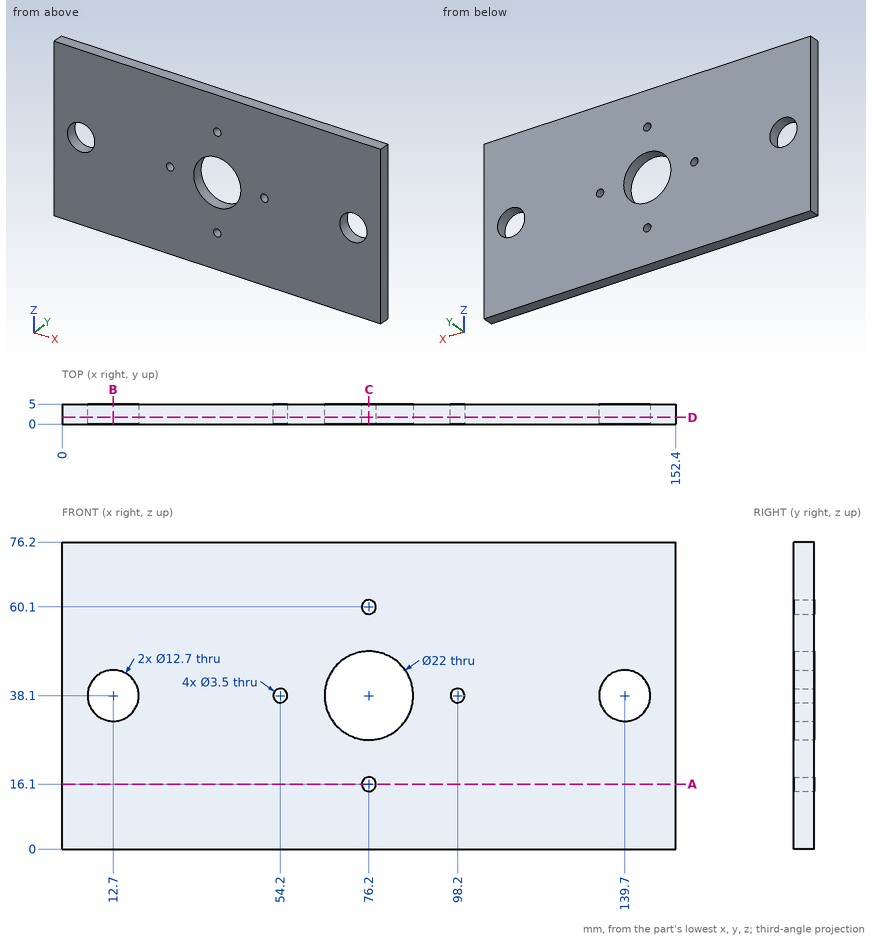
Input: dimensioned drawing with shaded views. Units: mm. Origin: part minimum x, y, z. Coordinates: 2 decimals unless noted, no trailing zeros. Order: outer loops, then holes, each group sorted by start corner. A loop starts at its lowest first (then second) coordinate and runs counter-clockwise, first axis right, second up. Notation, with made-up numbers: (-36.5, 70.25) -> (7.5, 70.25) arc R23 cw to (7.5, 91.25) -> close; hole circle Ø11 at (25.5, 30). An arc over 180 degrees is marked (long way). Use CSV: the item, a comma, the result in double quotes.
1) Section B-B on x = 12.7. Output: boundary loops of the cut face in (y, z), then the cut area to 4 significant figures.
Findings:
outline,"(0, 0) -> (5, 0) -> (5, 31.75) -> (0, 31.75) -> close; (0, 44.45) -> (5, 44.45) -> (5, 76.2) -> (0, 76.2) -> close"
area,"317.5 mm^2"
2) Line query: line 1 (Z direction, x = 98.2, y = 3.35); line 2 (X direction, y = 4.8, z = 41); line 3 (Z direction, x = 12.7, y = 1.65). Output: solid intervals per line, ascending.
Findings:
line 1,"z = 0 to 36.35, 39.85 to 76.2"
line 2,"x = 0 to 7.05, 18.35 to 65.59, 86.81 to 134.05, 145.35 to 152.4"
line 3,"z = 0 to 31.75, 44.45 to 76.2"
3) Pin query (flat end, axial travel): pin 1 Ø1 at (x, z) = (109, 56) entering from -Y; pin 2 Ø2 at (x, z) = (54.2, 38.1) entering from -Y. Return the tip coordinate at first contact, or that it passes through.
Findings:
pin 1,"stops at y = 0"
pin 2,"passes through"
4) Section C-C on x = 76.2. Output: boundary loops of the cut face in (y, z), then the cut area to 3 significant figures.
Findings:
outline,"(0, 0) -> (5, 0) -> (5, 14.35) -> (0, 14.35) -> close; (0, 17.85) -> (5, 17.85) -> (5, 27.1) -> (0, 27.1) -> close; (0, 49.1) -> (5, 49.1) -> (5, 58.35) -> (0, 58.35) -> close; (0, 61.85) -> (5, 61.85) -> (5, 76.2) -> (0, 76.2) -> close"
area,"236 mm^2"
5) Section A-A on z = 16.1. Output: boundary loops of the cut face in (x, y).
Findings:
outline,"(0, 0) -> (74.45, 0) -> (74.45, 5) -> (0, 5) -> close; (77.95, 0) -> (152.4, 0) -> (152.4, 5) -> (77.95, 5) -> close"
6) Section D-D on y = 1.65. Output: boundary loops of the cut face in (x, z).
Findings:
outline,"(0, 0) -> (152.4, 0) -> (152.4, 76.2) -> (0, 76.2) -> close; hole circle Ø12.7 at (12.7, 38.1); hole circle Ø3.5 at (54.2, 38.1); hole circle Ø22 at (76.2, 38.1); hole circle Ø3.5 at (76.2, 16.1); hole circle Ø3.5 at (76.2, 60.1); hole circle Ø3.5 at (98.2, 38.1); hole circle Ø12.7 at (139.7, 38.1)"
